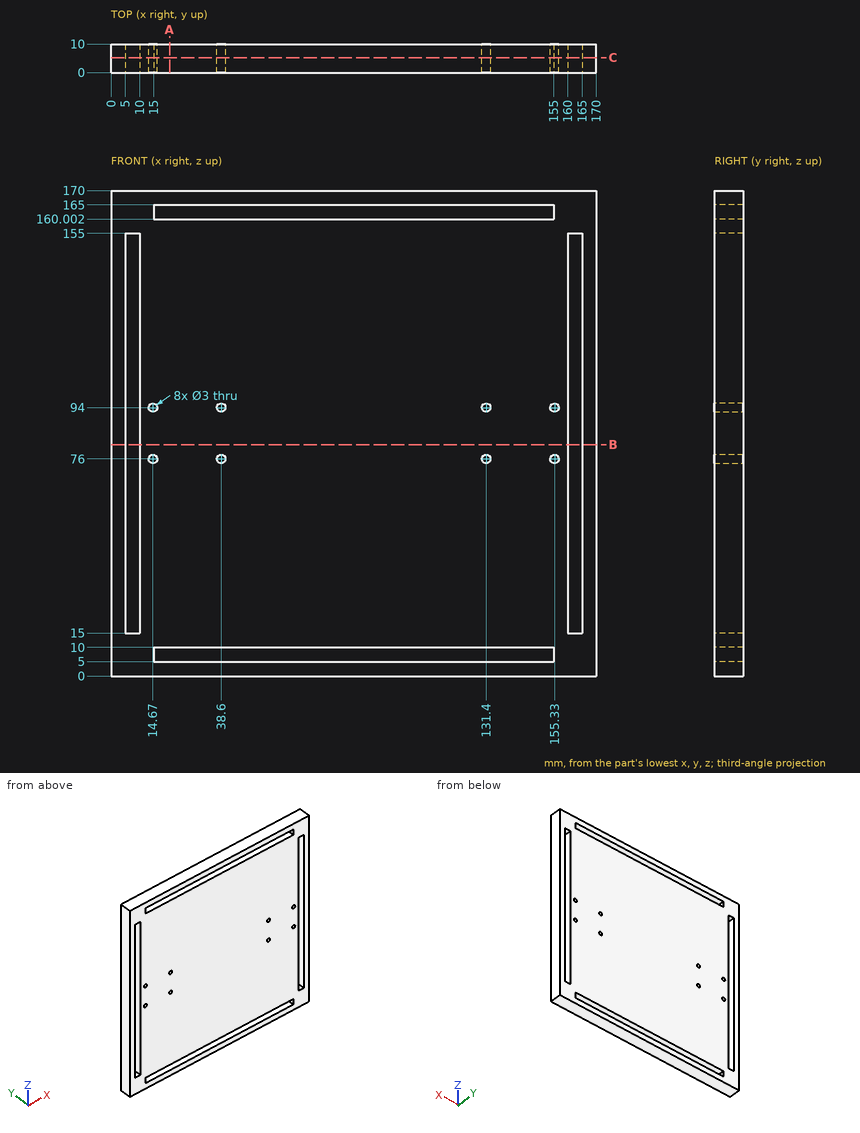
Answer from the drawing. Dimensions are ordinates in mm from the lowest x, y and z of the part. Round coordinates to 2 decimals unless told otherwise and drop trailing zeros. Loops run counter-clockwise (first coordinate to the right, second up) from the corner with the lowest first, then second, coordinate; pieces in that order, holes last. Notation, with made-up numbers: (85, -1) - (133, -1) arc R15 ccw to (133, 19) - close; hole circle Ø1 at (85, 87). An arc over 180 degrees is marked (long way). One line per item, written item: value.
Q1. Find section A-A on x = 20.5. Give the vertices of the cut face in (y, z).
Check values:
outline: (0, 0) - (10, 0) - (10, 5) - (0, 5) - close; (0, 10) - (10, 10) - (10, 160) - (0, 160) - close; (0, 165) - (10, 165) - (10, 170) - (0, 170) - close
Q2. Find section C-C on y = 5.25. State how many separate pieces and enclosed holes the cut face has, and give its area (3 significant figures).
Check values:
separate pieces: 1
enclosed holes: 12
area: 26,000 mm2
Q3. Find section B-B on z = 81. Give the vertices of the cut face in (x, y), and give its area (3 significant figures).
Check values:
outline: (0, 0) - (5, 0) - (5, 10) - (0, 10) - close; (10, 0) - (160, 0) - (160, 10) - (10, 10) - close; (165, 0) - (170, 0) - (170, 10) - (165, 10) - close
area: 1,600 mm2
Q4. Straight lines are drawn through the part: probe 1 along X at (y, z) = (1, 32); probe 2 along Z at (x, y) = (155.33, 5). For each, find the intervals that lie inside material, in ascending order.
Check values:
probe 1: 0 to 5, 10 to 160, 165 to 170
probe 2: 0 to 74.5, 77.5 to 92.5, 95.5 to 170
Q5. This flat-tipped pin is pushed along its axis until it touches: pin 1 Ø2.5 at (x, z) = (38.6, 76) entering from +Y. Where does it stop, or does it pass through?
Check values:
pin 1: through
